```python
from build123d import *

# Parameters (mm, degrees)
F0_W     = 76.2
F0_H     = 19.05
F0_R     = 4.572
F1_DEPTH = 6.35
F2_SIZE  = 6.35
F3_SIZE  = 6.35


with BuildPart() as f1:
    # F0 (on Front) → F1 (new body)
    with BuildSketch(Plane.XZ):
        with Locations((7.15868, 0.127)):
            Rectangle(F0_W, F0_H)
        with Locations((-21.79732, 0)):
            Circle(F0_R, mode=Mode.SUBTRACT)
        with Locations((36.11468, 0)):
            Circle(F0_R, mode=Mode.SUBTRACT)
    extrude(amount=F1_DEPTH)

    # F2
    f2_edges = [f1.edges().sort_by_distance(p)[0] for p in [
        (-30.94132, -3.175, 9.652),
        (45.25868, -3.175, 9.652),
        (45.25868, -3.175, -9.398),
    ]]
    chamfer(f2_edges, length=F2_SIZE)

    # F3
    f3_edges = [f1.edges().sort_by_distance(p)[0] for p in [
        (-30.94132, -3.175, -9.398),
    ]]
    chamfer(f3_edges, length=F3_SIZE)


solid = f1.part
```
Geometry check sheet. Reference: the model listing, model coordinates, mm. Give positions to 0.01 mm unless a question says otherwise; leave off trailing zeros. Order: outer loops, then holes, each group sorted by start corner. A loop starts at its lowest first (then second) coordinate and runs counter-clockwise, first axis right, second up. Notation, with made-up numbers: (28.25, -34.5) - (80.25, -34.5) arc R17 cw to (80.25, -18.5) - close; hole circle Ø7 at (-23.75, -33). An arc over 180 degrees is marked (long way). Write item = value, one per line. Start each with the question number.
1) Scan lines: L1, parallel to X at y = -0.75, z = -3.5; L2, parallel to X at y = -5.5, z = 3.75; L3, parallel to Z at x = -18, y = -5. Record each from-to range of solid material in increasing order.
2) Section check A-A (y = -2.5). Enter the section's corners in (x, z), then the cut area to 3 significant figures.
3) Section check C-C (x = 35). Enter the section's corners in (y, z), then the cut area to 3 significant figures.
4) Gauge pin test, flat end, axial feed: pin 1 Ø1.5 at (y, z) = (-3.5, 7.5) entering from +X. Record the tip position at first contact, or that the pin passes through.
5) Section check B-B (z = 0). Enter the section's corners in (x, y), then the cut area to 3 significant figures.
6) Section check D-D (x = -22.5). Enter the section's corners in (y, z), then the cut area to 3 significant figures.
7) Draft check along Z on faces 1 (the cylindrical face through (-17.574, -3.131, -1.751)), 2 (the flat face through (42.13, -3.13, 6.43)), 3 (the flat face through (45.259, -3, 0)). Enter one of: released by +Z, released by -Z, zero draft, split by the parting line, or undercut.
Geometry check:
q1.L1 = -30.49 to -24.74, -18.86 to 33.17, 39.06 to 44.81
q1.L2 = -30.49 to -24.41, -19.18 to 33.5, 38.73 to 44.81
q1.L3 = -9.4 to -2.55, 2.55 to 9.65
q2.outline = (-30.94, -3.05) - (-24.59, -9.4) - (38.91, -9.4) - (45.26, -3.05) - (45.26, 3.3) - (38.91, 9.65) - (-24.59, 9.65) - (-30.94, 3.3) - close; hole circle Ø9.14 at (-21.8, 0); hole circle Ø9.14 at (36.11, 0)
q2.area = 1,240 mm2
q3.outline = (-6.35, -9.4) - (0, -9.4) - (0, -4.43) - (-6.35, -4.43) - close; (-6.35, 4.43) - (0, 4.43) - (0, 9.65) - (-6.35, 9.65) - close
q3.area = 64.7 mm2
q4.pin_1 = 41.81
q5.outline = (-30.94, -6.35) - (-26.37, -6.35) - (-26.37, 0) - (-30.94, 0) - close; (-17.23, -6.35) - (31.54, -6.35) - (31.54, 0) - (-17.23, 0) - close; (40.69, -6.35) - (45.26, -6.35) - (45.26, 0) - (40.69, 0) - close
q5.area = 368 mm2
q6.outline = (-6.35, -9.4) - (0, -9.4) - (0, -4.52) - (-6.35, -4.52) - close; (-6.35, 4.52) - (0, 4.52) - (0, 9.65) - (-6.35, 9.65) - close
q6.area = 63.6 mm2
q7.face_1 = undercut
q7.face_2 = released by +Z
q7.face_3 = zero draft
